For this review, take the finished solid that the model builds, in its own axes (mm). Coordinates: 2 decimals unless noted, no trailing zeros. Loops run counter-clockwise (first coordinate to the right, second up) from the corner with the lowest first, then second, coordinate; pieces in that order, holes last. Notation, with made-up numbers: (22.5, 22) - (80.5, 22) arc R16 cw to (80.5, 44) - close; hole circle Ø5 at (-22, 7.5). An arc over 180 degrees is marked (long way). Use one line per item in the form item = value. Start each with the question number.
1. Add section D-D on y = 5.5. Give the boundary of the cut face in (x, z), and give its area (3 significant figures).
2. Add section A-A on z = 1.9. Give the boundary of the cut face in (x, y).
3. Add section C-C on z = 0.4. Give the boundary of the cut face in (x, y).
4. For pin 1 Ø1.5 at (x, y) = (2, -6.5) entering from +Z; pin 2 Ø1.5 at (x, z) = (-2, 1.5) entering from +Y, all flat-tipped, find the tip position at first contact; note any pin that passes through.
5. To check wall thickness, follow probe 1 along Y at (x, z) = (-1.75, 2.6); probe 2 along Z at (x, y) = (1, 10); probe 3 along Y at (x, z) = (1, 1.4). State the ranges of each line that lie inside material, in increasing order.
6. Add section B-B on y = -2. Give the boundary of the cut face in (x, z), and give its area (3 significant figures).
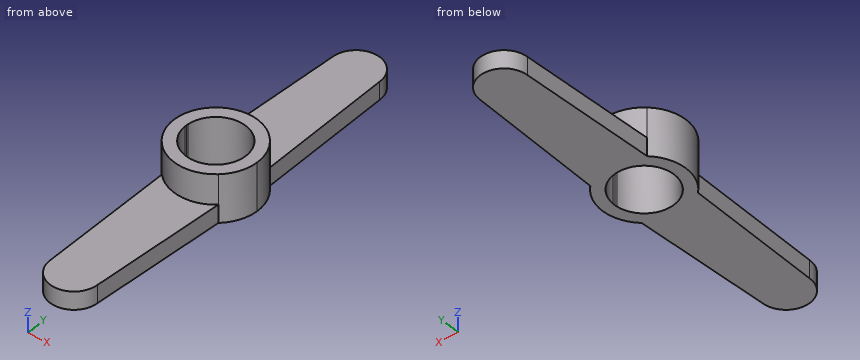
```python
from build123d import *

# Parameters (mm, degrees)
BOSS_EXTRU_1_DEPTH = 4
ESQUISSE1_3_R      = 2
BOSS_EXTRU_2_DEPTH = 1.5


with BuildPart() as part:
    # Esquisse1 → Boss.-Extru.1 (new body)
    with BuildSketch(Plane.XY):
        with BuildLine():
            Line((-2.42213609, 2.526510788), (-2.495255529, 0.153947543))
            ThreePointArc((-2.495255529, 0.153947543), (-0.024445902, 2.499880477), (2.491767789, 0.202714787))
            Line((2.491767789, 0.202714787), (2.396407287, 2.550927696))
            ThreePointArc((2.396407287, 2.550927696), (-0.017735252, 3.499955066), (-2.42213609, 2.526510788))
        make_face()
        with BuildLine():
            ThreePointArc((2.491767789, 0.202714787), (2.497941099, 0.101440936), (2.5, 0))
            ThreePointArc((2.5, 0), (2.497941099, -0.101440936), (2.491767789, -0.202714787))
            Line((2.491767789, -0.202714787), (2.396407287, -2.550927696))
            ThreePointArc((2.396407287, -2.550927696), (3.212275323, -1.389707612), (3.5, 0))
            ThreePointArc((3.5, 0), (3.212275323, 1.389707612), (2.396407287, 2.550927696))
            Line((2.396407287, 2.550927696), (2.491767789, 0.202714787))
        make_face()
        with BuildLine():
            ThreePointArc((2.491767789, -0.202714787), (-0.024445902, -2.499880477), (-2.495255529, -0.153947543))
            Line((-2.495255529, -0.153947543), (-2.42213609, -2.526510788))
            ThreePointArc((-2.42213609, -2.526510788), (-0.017735252, -3.499955066), (2.396407287, -2.550927696))
            Line((2.396407287, -2.550927696), (2.491767789, -0.202714787))
        make_face()
        with BuildLine():
            ThreePointArc((-2.495255529, -0.153947543), (-2.498813601, -0.077010317), (-2.5, 0))
            ThreePointArc((-2.5, 0), (-2.498813601, 0.077010317), (-2.495255529, 0.153947543))
            Line((-2.495255529, 0.153947543), (-2.42213609, 2.526510788))
            ThreePointArc((-2.42213609, 2.526510788), (-3.5, 0), (-2.42213609, -2.526510788))
            Line((-2.42213609, -2.526510788), (-2.495255529, -0.153947543))
        make_face()
    extrude(amount=BOSS_EXTRU_1_DEPTH)

    # Esquisse1_3 → Boss.-Extru.2 (add)
    with BuildSketch(Plane.XY):
        with BuildLine():
            Line((-2.068537469, 14), (-2.42213609, 2.526510788))
            ThreePointArc((-2.42213609, 2.526510788), (-0.017735252, 3.499955066), (2.396407287, 2.550927696))
            Line((2.396407287, 2.550927696), (1.931462531, 14))
            ThreePointArc((1.931462531, 14), (-0.068537469, 12), (-2.068537469, 14))
        make_face()
        with BuildLine():
            ThreePointArc((1.931462531, 14), (-0.068537469, 16), (-2.068537469, 14))
            Line((-2.068537469, 14), (1.931462531, 14))
        make_face()
        with BuildLine():
            Line((1.931462531, 14), (-2.068537469, 14))
            ThreePointArc((-2.068537469, 14), (-0.068537469, 12), (1.931462531, 14))
        make_face()
        with BuildLine():
            ThreePointArc((2.396407287, -2.550927696), (-0.017735252, -3.499955066), (-2.42213609, -2.526510788))
            Line((-2.42213609, -2.526510788), (-2.068537469, -14))
            ThreePointArc((-2.068537469, -14), (-0.068537469, -12), (1.931462531, -14))
            Line((1.931462531, -14), (2.396407287, -2.550927696))
        make_face()
        with Locations((-0.068537469, -14)):
            Circle(ESQUISSE1_3_R)
    extrude(amount=BOSS_EXTRU_2_DEPTH)


solid = part.part
```
Conclusion:
q1.outline = (-2.33, 0) - (2.28, 0) - (2.28, 1.5) - (-2.33, 1.5) - close
q1.area = 6.91 mm^2
q2.outline = circle Ø7 at (0, 0); hole circle Ø5 at (0, 0)
q3.outline = (-2.42, -2.53) - (-2.07, -14) arc R2 ccw to (1.93, -14) - (2.4, -2.55) arc R3.5 ccw to (2.4, 2.55) - (1.93, 14) arc R2 ccw to (-2.07, 14) - (-2.42, 2.53) arc R3.5 ccw to start; hole circle Ø5 at (0, 0)
q4.pin_1 = 1.5
q4.pin_2 = 15.61
q5.probe_1 = -3.03 to -1.79, 1.79 to 3.03
q5.probe_2 = 0 to 1.5
q5.probe_3 = -15.69 to -2.29, 2.29 to 15.69
q6.outline = (-2.87, 0) - (-1.5, 0) - (-1.5, 4) - (-2.87, 4) - close; (1.5, 0) - (2.87, 0) - (2.87, 4) - (1.5, 4) - close
q6.area = 11.0 mm^2
